Design review of the part built by this model. Coordinates are the model's own, in mm. Give positions to 0.01 mm unless a question says otherwise; leave off trailing zeros. Loops run counter-clockwise (first coordinate to the right, second up) from the corner with the lowest first, then second, coordinate; pieces in that order, holes last. Notation, with made-up numbers: M 82.5,-34 L 116.5,-34 A21 ccw 116.5,1 Z; hole C -1,63.25 d2. An arc over 180 degrees is marked long. Answer as CSV lines item,"result".
Autodesk Fusion 360 part; units mm, degrees
sketch "Sketch1" plane through (0, 0, 0) normal (0, 0, 1) x (1, 0, 0)
  circle A0 centre (0, 0) radius 40
  circle A1 centre (0, 0) radius 28
  circle A2 centre (0, 0) radius 11
  circle A3 centre (28, 0.0227) radius 7
  circle A4 centre (19.7829, 19.815) radius 7
  circle A5 centre (-0.0227, 28) radius 7
  circle A6 centre (-19.815, 19.7829) radius 7
  circle A7 centre (-28, -0.0227) radius 7
  circle A8 centre (-19.7829, -19.815) radius 7
  circle A9 centre (0.0227, -28) radius 7
  circle A10 centre (19.815, -19.7829) radius 7
  dimension "d1" = 80
  dimension "d2" = 56
  dimension "d3" = 22
  dimension "d4" = 14
  dimension "d6" = 360
extrude "Extrude1" add sketch "Sketch1" along normal blind 20 contours A0 | A1 A3 A4 A5 A6 A7 A8 A9 A10
1. To check wall thickness, follow L1, parallel to Y at x = 0, z = 9; L2, parallel to X at y = -0.5, z = 16.25; L3, parallel to Y at x = 25, z = 1.25. State the ranges of each line that lie inside material, in increasing order. Write a range as [from, to].
Answer block:
L1,"[-40, -35], [-21, -11], [11, 21], [35, 40]"
L2,"[-40, -34.98], [-21.02, -10.99], [10.99, 21.02], [34.98, 40]"
L3,"[-31.22, -24.49], [-15.08, -6.3], [6.35, 15.15], [24.48, 31.22]"
2. The part is to be moulded in two halves that separate along Y. For faces 1 (the cylindrical face through (-21.323, -2.125, 9.86)), 2 (the cylindrical face through (-8.67, 39.05, 9.86)), 3 (the flat face through (8, -8, 20)), say which applies: pulls with the +Y half, pulls with the -Y half, needs draft (parallel to the pull), parting line crosses it, or undercut.
Answer block:
face 1,"undercut"
face 2,"parting line crosses it"
face 3,"needs draft"
3. For P1, Ø11, axis at x = -19.78, y = -19.82, coming from the +Z side; P2, Ø6, axis at y = 30, z = 3.5, coming from the +X side; P3, Ø6, axis at x = -28, z = 15, coming from the -Y side (3 decimals); P4, Ø12, axis at y = -12, z = 7, coming from the -X side, all flat-tipped, find the tip position at first contact; note any pin that passes through.
Answer block:
P1,"through"
P2,"x = 29.51"
P3,"y = -31.225"
P4,"x = -39.55"
4. We need section C-C, the plane y = 1. Write out the cut boundary in (x, z), plus the area to 3 significant figures.
Answer block:
outline,"M -39.99,0 L -34.92,0 L -34.92,20 L -39.99,20 Z; M -21.08,0 L -10.95,0 L -10.95,20 L -21.08,20 Z; M 10.95,0 L 21.07,0 L 21.07,20 L 10.95,20 Z; M 34.93,0 L 39.99,0 L 39.99,20 L 34.93,20 Z"
area,"607 mm²"
5. We need section A-A, the plane y = -28. Write out the cut boundary in (x, z), plus the area to 3 significant figures.
Answer block:
outline,"M -28.57,0 L -6.98,0 L -6.98,20 L -28.57,20 Z; M 7.02,0 L 28.57,0 L 28.57,20 L 7.02,20 Z"
area,"863 mm²"
6. We need section D-D, the plane x = -4.5. Write out the cut boundary in (y, z), plus the area to 3 significant figures.
Answer block:
outline,"M -39.75,0 L -33.34,0 L -33.34,20 L -39.75,20 Z; M -22.66,0 L -10.04,0 L -10.04,20 L -22.66,20 Z; M 10.04,0 L 22.62,0 L 22.62,20 L 10.04,20 Z; M 33.38,0 L 39.75,0 L 39.75,20 L 33.38,20 Z"
area,"759 mm²"
